Autodesk Inventor part; units mm, degrees
ref_plane "YZ Plane" through (0, 0, 0) normal (1, 0, 0) x (0, 1, 0)
ref_plane "XZ Plane" through (0, 0, 0) normal (0, 1, 0) x (-1, 0, 0)
ref_plane "XY Plane" through (0, 0, 0) normal (0, 0, 1) x (1, 0, 0)
sketch "Szkic5" plane through (0, 0, 0) normal (0, 0, 1) x (1, 0, 0)
  line L0 (-18.8, 0) -> (18.8, 0)
  line L1 (0, 0) -> (0, 20.8) construction
  arc A0 (18.8, 20.8) -> (-18.8, 20.8) centre (0, 20.8) ccw
  line L2 (-18.8, 0) -> (-18.8, 20.8)
  line L3 (18.8, 0) -> (18.8, 20.8)
  circle A1 centre (0, 20.8) radius 15.5 construction
  line L4 (0, 27.8) -> (0, 13.8) construction
  line L5 (0, 27.8) -> (0, 13.8) construction
  line L6 (-6.6, 27.8) -> (-6.6, 13.8)
  line L7 (6.6, 13.8) -> (6.6, 27.8)
  arc A2 (6.6, 27.8) -> (-6.6, 27.8) centre (0, 27.8) ccw
  arc A3 (-6.6, 13.8) -> (6.6, 13.8) centre (0, 13.8) ccw
  point P0 (-15.5, 20.8)
  point P1 (0, 20.8)
  dimension "d35" = 31
  dimension "d26" = 37.6
  dimension "d27" = 20.8
  dimension "d28" = 37.6
  dimension "d46" = 14
  dimension "d47" = 13.2
extrude "Wyciągnięcie proste4" add sketch "Szkic5" against normal blind 2 contours L2 A0 L3 L0 | A2 L7 A3 L6
sketch "Szkic6" plane through (18.8, 0, 0) normal (1, 0, 0) x (0, 0, -1)
  line L0 (2, 0) -> (2, 20.8)
  line L1 (2, 0) -> (51.2, 0)
  line L2 (51.2, 0) -> (51.2, 2)
  line L3 (51.2, 2) -> (2, 2)
  line L4 (2, 2) -> (2, 0)
  point P0 (0, 0)
  dimension "d31" = 49.2
  dimension "d32" = 2
extrude "Wyciągnięcie proste5" add sketch "Szkic6" against normal up to surface (37.6 mm away)
hole "Otwór2" at (-15.5, 20.8, 0) direction (0, 0, -1) diameter 3.3 end through all
pattern_circular "Szyk kołowy2" count 6 over 360 about axis through (0, 20.8, 0) along (0, 0, -1) of "Otwór2"
extrude "Wyciągnięcie proste6" cut sketch "Szkic5" against normal through all contours A2 L7 A3 L6
sketch "Szkic7" plane through (18.8, 2, -2) normal (0, 1, 0) x (1, 0, 0)
  line L0 (-18.8, -2) -> (-18.8, 44.5) construction
  line L1 (-34.4, 44.5) -> (-3.2, 44.5) construction
  dimension "d50" = 31.2
  dimension "d51" = 46.5
hole "Otwór3" at (-15.6, 2, -46.5) direction (0, -1, 0) diameter 3.2 end through all
pattern_linear "Szyk prostokątny1" count 7 spacing 6.4 along (0, 0, 1) of "Otwór3"
mirror "Odbij1" about plane through (0, 0, 0) normal (1, 0, 0) of "Otwór3", "Szyk prostokątny1"
fillet "Zaokrąglenie1" radius 4 2 edges at (18.8, 1, -51.2) (-18.8, 1, -51.2)
fillet "Zaokrąglenie2" radius 2 1 edges at (0, 0, 0)
properties part number "bepf_podwozie_lacznik_silnika" material "Aluminium 6061"
Input: part model. Units: mm. Frame: model coordinates. A direction names the side the tool comes from. Round coordinates to 2 decimals unless told otherwise and drop trailing zeros. Write each loop counter-clockwise with the first axis right and the second up, starting at its lowest first coordinate (ties: lowest second). Pieces come first, ordered by that corner, then holes.
1) Cut plane C-C (y = 20). Return the cut outline in (x, z), then the cut area to 3 significant figures.
2) Draft query along Z for faces 3 (the flat face through (-6.6, 21, -1)), 4 (the flat face through (8, 17, -2)), 5 (the cylindrical face through (-14.99, 0.99, -32.22)). Return one class per face: pulls with the +Z half, pulls with the -Z half, needs draft (parallel to the pull), parting line crosses it, or undercut.
3) Cut plane D-D (x = -7.75). Return the cut outline in (y, z), then the cut area to 3 significant figures.
4) Cut plane B-B (x = 0). Return the cut outline in (y, z).
5) Contact query for flat-ended pins moving along their axis: P1, Ø2, axis at x = -7.75, y = 34.22, coming from the -Z side; P2, Ø3.5, axis at x = -15.6, z = -14.5, coming from the +Y side; P3, Ø4, axis at x = -7.5, y = 30.5, coming from the -Z side. Output: stop coordinate, or through.
6) Cut plane A-A (z = -27.3). Return the cut outline in (x, y), then the cut area to 3 significant figures.
7) Ray query, L1, parallel to X at y = 1.1, z = -40.1; L2, parallel to Y at x = -11, z = -26.5; L3, parallel to Z at x = -14, y = 13. Return the intervals inside material, ascending.
8) Reachability of faces 1 (the cylindrical face through (15.53, 0.99, -16.1)), 2 (the cylindrical face through (0.1, 34.4, -1)) from +Z, -Z, +X, -X, +Y, -Y: full face, straight path, thin tool, end or side. Return the list, or none.
Geometry says:
1. outline: (-18.8, -2) - (-16.94, -2) - (-16.94, 0) - (-18.8, 0) - close; (-14.06, -2) - (-6.6, -2) - (-6.6, 0) - (-14.06, 0) - close; (6.6, -2) - (14.06, -2) - (14.06, 0) - (6.6, 0) - close; (16.94, -2) - (18.8, -2) - (18.8, 0) - (16.94, 0) - close
1. area: 37.3 mm2
2. face 3: needs draft
2. face 4: pulls with the -Z half
2. face 5: undercut
3. outline: (0, -51.2) - (2, -51.2) - (2, -2) - (5.73, -2) - (5.73, 0) - (2, 0) arc R2 ccw to (0, -2) - close; (9.03, -2) - (32.57, -2) - (32.57, 0) - (9.03, 0) - close; (35.87, -2) - (37.93, -2) - (37.93, 0) - (35.87, 0) - close
3. area: 160 mm2
4. outline: (0, -51.2) - (2, -51.2) - (2, -2) - (7.2, -2) - (7.2, 0) - (2, 0) arc R2 ccw to (0, -2) - close; (34.4, -2) - (39.6, -2) - (39.6, 0) - (34.4, 0) - close
5. P1: passes through
5. P2: stops at y = 2
5. P3: stops at z = -2
6. outline: (-18.8, 0) - (-17.2, 0) - (-17.2, 2) - (-18.8, 2) - close; (-14, 0) - (14, 0) - (14, 2) - (-14, 2) - close; (17.2, 0) - (18.8, 0) - (18.8, 2) - (17.2, 2) - close
6. area: 62.4 mm2
7. L1: x = -18.8 to -17.2, -14 to 14, 17.2 to 18.8
7. L2: y = 0 to 2
7. L3: z = -2 to 0
8. face 1: +Y, -Y
8. face 2: +Z, -Z
